Autodesk Inventor part; units mm, degrees
ref_plane "YZ Plane" through (0, 0, 0) normal (1, 0, 0) x (0, 1, 0)
ref_plane "XZ Plane" through (0, 0, 0) normal (0, 1, 0) x (-1, 0, 0)
ref_plane "XY Plane" through (0, 0, 0) normal (0, 0, 1) x (1, 0, 0)
sketch "Schizzo9" plane through (0, 0, 0) normal (0, 0, 1) x (1, 0, 0)
  line L0 (-50, 5) -> (50, 5)
  line L1 (50, 5) -> (50, -5)
  line L2 (50, -5) -> (-50, -5)
  line L3 (-50, -5) -> (-50, 5)
  line L4 (-50, 5) -> (50, -5) construction
  line L5 (50, 5) -> (-50, -5) construction
  point P0 (0, 0)
  dimension "d87" = 100
  dimension "d88" = 10
extrude "Piano6" add sketch "Schizzo9" along normal blind 1
sketch "Schizzo19" plane through (-50, 6, 2) normal (0, 1, 0) x (-1, 0, 0)
  line L0 (-100, 0) -> (0, 0)
  line L1 (0, 0) -> (0, 6)
  line L2 (0, 6) -> (-100, 6)
  line L3 (-100, 6) -> (-100, 0)
edge flange "Flangia9" height 8 angle 90 thickness 1 bend radius 1 thickness toward (0, 1, 0) relief tear relief width 1 relief depth 0.5 edges at (0, 5, 1) wall of the first edge with corners at (50, 6, 2) (-50, 6, 2) (-50, 6, 8) (50, 6, 8)
bend "Piega (Bend)9"
corner "Angolo9"
sketch "Schizzo20" plane through (-51, 5, 2) normal (-1, 0, 0) x (0, -1, 0)
  line L0 (0, 6) -> (0, 0)
  line L1 (0, 0) -> (10, 0)
  line L2 (10, 0) -> (10, 6)
  line L3 (10, 6) -> (0, 6)
edge flange "Flangia10" height 12 angle 90 thickness 1 bend radius 1 thickness toward (-1, 0, 0) relief tear relief width 1 relief depth 0.5 edges at (-50, 6, 5) wall of the first edge with corners at (-51, 5, 8) (-51, 5, 2) (-51, -5, 2) (-51, -5, 8)
bend "Piega (Bend)10"
corner "Angolo10"
sketch "Schizzo21" plane through (0, 0, 1) normal (0, 0, 1) x (1, 0, 0)
  line L0 (50, 5) -> (50, -5)
  point P0 (0, 0)
  point P1 (40, 0)
  point P2 (50, 0)
  dimension "d202" = 10
hole "Foro7" at (40, 0, 1) direction (0, 0, -1) diameter 5 end through all
fillet "Arrotondamento angolo7" radius 2 5 edges at (50, 6.5, 8) (50, -5, 0.5) (-50, -5, 0.5) (-51.5, -5, 2) (-51.5, -5, 8)
sketch "Schizzo22" plane through (-52, 5, 2) normal (-1, 0, 0) x (0, 0, 1)
  line L0 (6, 0) -> (6, -8)
  line L1 (4, -10) -> (2, -10)
  point P0 (-2, -5)
  point P1 (3, -5)
  point P2 (3, -10)
hole "Foro8" at (-52, 0, 5) direction (1, 0, 0) diameter 5 end through all
equation "\"d208\" = Spessore"
equation "\"d217\" = Spessore"
equation "\"d89\" = Spessore"
equation "\"d182\" = LarghezzaScaricoPiega"
equation "\"d183\" = ProfonditàScaricoPiega"
equation "\"d184\" = ResiduoMinimo"
equation "\"d185\" = RaggioTransizione"
equation "\"d188\" = RaggioPiega"
equation "\"d189\" = DimensioniScaricoAngolo"
equation "\"d190\" = DimensioneGioco"
equation "\"d191\" = Dimensione_raggio_Jacobi"
equation "\"d192\" = LarghezzaScaricoPiega"
equation "\"d193\" = ProfonditàScaricoPiega"
equation "\"d194\" = ResiduoMinimo"
equation "\"d195\" = RaggioTransizione"
equation "\"d198\" = RaggioPiega"
equation "\"d199\" = DimensioniScaricoAngolo"
equation "\"d200\" = DimensioneGioco"
equation "\"d201\" = Dimensione_raggio_Jacobi"
equation "\"RaggioPiega\" = Spessore"
equation "\"LarghezzaScaricoPiega\" = Spessore"
equation "\"ProfonditàScaricoPiega\" = 0.5 * Spessore"
equation "\"DimensioniScaricoAngolo\" = 4 * Spessore"
equation "\"ResiduoMinimo\" = 2 * Spessore"
equation "\"RaggioTransizione\" = RaggioPiega"
equation "\"Dimensione_raggio_Jacobi\" = RaggioPiega"
equation "\"DimensioneGioco\" = Spessore"
properties part number "Lamiera pistone scarico"
Check sheet for the modelled part. Datum: model origin and axes. Units: mm. A direction names the side the tool comes from. Round coordinates to 2 decimals unless told otherwise and drop trailing zeros. Write each loop counter-clockwise with the first axis right and the second up, starting at its lowest first coordinate (ties: lowest second). Pieces come first, ordered by that corner, then holes. Notation, with made-up numbers: (42, 5.5) -> (57, 5.5) arc R15 cw to (57, 19.5) -> close; hole circle Ø3 at (31.5, 84). An arc over 180 degrees is marked (long way). Put each result on its own line as item: value.
(1) Sectioned sample at C-C (x = 5). Enter the section's corners in (y, z), plus the area to 3 significant figures.
Values found:
outline: (-5, 0) -> (5, 0) arc R2 ccw to (7, 2) -> (7, 8) -> (6, 8) -> (6, 2) arc R1 cw to (5, 1) -> (-5, 1) -> close
area: 18.4 mm^2
(2) Sectioned sample at A-A (y = 0). Enter the section's corners in (x, z), plus the area to 3 significant figures.
Values found:
outline: (-52, 2) -> (-51, 2) -> (-51, 2.5) -> (-52, 2.5) -> close; (-52, 7.5) -> (-51, 7.5) -> (-51, 8) -> (-52, 8) -> close; (-50, 0) -> (37.5, 0) -> (37.5, 1) -> (-50, 1) -> close; (42.5, 0) -> (50, 0) -> (50, 1) -> (42.5, 1) -> close
area: 96.0 mm^2
(3) Sectioned sample at B-B (z = 5). Enter the section's corners in (x, y).
Values found:
outline: (-52, -5) -> (-51, -5) -> (-51, -2.5) -> (-52, -2.5) -> close; (-52, 2.5) -> (-51, 2.5) -> (-51, 5) arc R1 cw to (-50, 6) -> (50, 6) -> (50, 7) -> (-50, 7) arc R2 ccw to (-52, 5) -> close
(4) Go/stop test with flat-tipped pins: pin 1 Ø0.6 at (y, z) = (2, 1) entering from -X; pin 2 Ø1 at (x, y) = (36, 0.5) entering from +Z; pin 3 Ø3 at (x, z) = (-2, 5) entering from -Y; pin 4 Ø4.5 at (y, z) = (0, 5) entering from +X. Record where each tip stops, or that it passes through.
Values found:
pin 1: stops at x = -50
pin 2: stops at z = 1
pin 3: stops at y = 6
pin 4: passes through
(5) Mould release check, pull along Y, two halves, no side actions. Record for faces 1 (the face through (-51.493, -0.751, 7.385)), 2 (the face through (-1, 7, 5)), 3 (the face through (49.4, -4.43, 0.51)), 4 (the face through (-2.2, 6.4, 8)): released by +Y, released by -Y, zero draft, split by the parting line, or undercut.
Values found:
face 1: undercut
face 2: released by +Y
face 3: released by -Y
face 4: zero draft
(6) Tool access check on faces 5 (the face through (-51.5, 1.9, 2)), 6 (the face through (-1, 0, 1)), 7 (the face through (-51, 2.3, 3.6)). Record the directions out of +Z, -Z, +X, -X, +Y, -Y that give a thin tool (end or side, any length) a straight path to the whole face; none if there is none.
Values found:
face 5: -Z, -X, +Y, -Y
face 6: +Z, +X, -X, -Y
face 7: +Z, -Z, +X, -Y
(7) Material ranges on line 1 (X direction, y = 0, z = 0.55); line 2 (Z direction, x = -51.5, y = 0); line 3 (Y direction, x = -41, z = 6.5), recorded low to high.
Values found:
line 1: x = -50 to 37.5, 42.5 to 50
line 2: z = 2 to 2.5, 7.5 to 8
line 3: y = 6 to 7
